Here's how the part is built. I have some questions about the finished solid (model axes, mm). A direction names the side the tool comes from. Round coordinates to 2 decimals unless told otherwise and drop trailing zeros. Order: outer loops, then holes, each group sorted by start corner. A loop starts at its lowest first (then second) coordinate and runs counter-clockwise, first axis right, second up.
```python
from build123d import *

# Parameters (mm, degrees)
SKETCH_1_W          = 28
SKETCH_1_H          = 24
EXTRUDE_1_DEPTH     = 2
SKETCH_1_5_R        = 1.5
SKETCH_1_5_W        = 7
SKETCH_1_5_H        = 2
SKETCH_1_5_W_2      = 3
SKETCH_1_5_H_2      = 7
SKETCH_1_5_W_3      = 16
SKETCH_1_5_W_4      = 6.6
CUT_EXTRUDE_1_DEPTH = 37.932370625


with BuildPart() as part:
    # Sketch 1 → Extrude 1 (new body)
    with BuildSketch(Plane(origin=(0, 0, 0), x_dir=(1, 0, 0), z_dir=(0, 1, 0))):
        with Locations((-14, -12)):
            Rectangle(SKETCH_1_W, SKETCH_1_H)
    extrude(amount=EXTRUDE_1_DEPTH)

    # Sketch 1_5 → Cut-Extrude 1 (cut, through all)
    with BuildSketch(Plane(origin=(0, 0, 0), x_dir=(1, 0, 0), z_dir=(0, 1, 0))):
        with Locations(Location((-25, -3, 0), (0, 0, 270))):
            Circle(SKETCH_1_5_R)
        with Locations(Location((-3, -3, 0), (0, 0, 270))):
            Circle(SKETCH_1_5_R)
        with Locations(Location((-25, -21, 0), (0, 0, 270))):
            Circle(SKETCH_1_5_R)
        with Locations(Location((-3, -21, 0), (0, 0, 270))):
            Circle(SKETCH_1_5_R)
        with Locations((-14.5, -21.8)):
            Rectangle(SKETCH_1_5_W, SKETCH_1_5_H)
        with Locations((-4.2, -11.5)):
            Rectangle(SKETCH_1_5_W_2, SKETCH_1_5_H_2)
        with Locations((-14.3, -3.7)):
            Rectangle(SKETCH_1_5_W_3, SKETCH_1_5_H)
        with Locations((-24.7, -14.7)):
            Rectangle(SKETCH_1_5_W_4, SKETCH_1_5_H)
        with Locations((-24.7, -8.5)):
            Rectangle(SKETCH_1_5_W_4, SKETCH_1_5_H)
        with Locations((-14.5, -19.4)):
            Rectangle(SKETCH_1_5_W_3, SKETCH_1_5_H)
    extrude(amount=CUT_EXTRUDE_1_DEPTH, mode=Mode.SUBTRACT)


solid = part.part
```
1. If we mould it in two halves opening along X, with no side actions, what happens to faces 1 (the flat face through (-25, 1, 13.7)), 2 (the flat face through (0, 1, 12)), 3 (the flat face through (-6.3, 1, 4)), 4 (the flat face through (-28, 1, 4))? For each: released by +X, released by -X, zero draft, split by the parting line, or undercut.
Evaluation:
face 1: zero draft
face 2: released by +X
face 3: undercut
face 4: released by -X
2. On a 3-axis mill with a long thin cutter (end or side, diameter ignored), from which of +Z, -Z, +X, -X, +Y, -Y can I reach the whole of each face in a straight line? I mean faces 5 (the flat face through (-5.7, 1, 12)), 6 (the flat face through (-25, 1, 9.5)), 7 (the flat face through (-14, 0, 12)). Say none if no direction works.
Evaluation:
face 5: +Y, -Y
face 6: -X, +Y, -Y
face 7: +Z, -Z, +X, -X, -Y
3. If we section it at C-C, the plane z = 12.75: Write out the boundary of the cut face in (x, y).
Evaluation:
outline: (-28, 0) - (-5.7, 0) - (-5.7, 2) - (-28, 2) - close; (-2.7, 0) - (0, 0) - (0, 2) - (-2.7, 2) - close
4. If we section it at A-A, the plane x = -3: Write out the boundary of the cut face in (y, z).
Evaluation:
outline: (0, 0) - (2, 0) - (2, 1.5) - (0, 1.5) - close; (0, 4.5) - (2, 4.5) - (2, 8) - (0, 8) - close; (0, 15) - (2, 15) - (2, 19.5) - (0, 19.5) - close; (0, 22.5) - (2, 22.5) - (2, 24) - (0, 24) - close
5. I need wall thicknesses on probe 1 along Z at (x, y) = (-3, 0.4); probe 2 along Z at (x, y) = (-8, 1); probe 3 along Z at (x, y) = (-15, 0.75). Which ranges of each line are inside material? Lowest first, please.
Evaluation:
probe 1: z = 0 to 1.5, 4.5 to 8, 15 to 19.5, 22.5 to 24
probe 2: z = 0 to 2.7, 4.7 to 18.4, 20.4 to 24
probe 3: z = 0 to 2.7, 4.7 to 18.4, 20.4 to 20.8, 22.8 to 24
6. If we section it at B-B, the plane y = 1.7: State how many separate pieces and enclosed holes the cut face has, and give its area (3 significant figures).
Evaluation:
separate pieces: 1
enclosed holes: 8
area: 518 mm2
7. If we section it at D-D, the plane x = -9.25: Write out the boundary of the cut face in (y, z), and give its area (3 significant figures).
Evaluation:
outline: (0, 0) - (2, 0) - (2, 2.7) - (0, 2.7) - close; (0, 4.7) - (2, 4.7) - (2, 18.4) - (0, 18.4) - close; (0, 20.4) - (2, 20.4) - (2, 24) - (0, 24) - close
area: 40.0 mm2
